Design review of the part built by this model. Coordinates are the model's own, in mm. A direction names the side the tool comes from. Coordinates: 2 decimals unless noted, no trailing zeros. Order: outer loops, then holes, each group sorted by start corner. A loop starts at its lowest first (then second) coordinate and runs counter-clockwise, first axis right, second up. Notation, with made-up numbers: M 55.25,78.5 L 100.25,78.5 A14 ccw 100.25,90.5 Z; hole C 34.5,44.25 d3. An arc over 180 degrees is marked long. Use CSV: the item, a comma, the result in double quotes.
```python
from build123d import *

# Parameters (mm, degrees)
FILLET1_R     = 2.5
CHAMFER1_SIZE = 1


with BuildPart() as part:
    # Sketch1 → Revolve1 (revolve)
    with BuildSketch(Plane.XY, mode=Mode.PRIVATE) as revolve1_sk:
        Polygon((0, 0), (251, 0), (251, 16), (206, 16), (206, 18.5), (170, 18.5), (170, 21), (70, 21), (70, 18.5), (45, 18.5), (45, 16), (0, 16), align=None)
    revolve(revolve1_sk.sketch.rotate(Axis((0, 0, 0), (1, 0, 0)), 90), axis=Axis((0, 0, 0), (1, 0, 0)))

    # Fillet1
    fillet1_edges = [part.edges().sort_by_distance(p)[0] for p in [
        (170, 0, -18.5),
        (70, 0, -18.5),
        (45, 0, -16),
        (206, 0, -16),
    ]]
    fillet(fillet1_edges, radius=FILLET1_R - 0.0001)  # a hair under: the kernel refuses the full size

    # Chamfer1
    chamfer1_edges = [part.edges().sort_by_distance(p)[0] for p in [
        (0, 0, -16),
        (251, 0, -16),
    ]]
    chamfer(chamfer1_edges, length=CHAMFER1_SIZE)


solid = part.part
```
(1) Add section C-C on x = 137.5. State the section outline as (y, z) points.
The answers:
outline,"C 0,0 d42"
(2) Clearance check with flat-ended pins moving along their axes: P1, Ø3, axis at x = 139, y = 9, coming from the +Z side; P2, Ø6, axis at x = 183, y = -12.5, coming from the +Z side; P3, Ø2, axis at x = 112, y = 11, coming from the -Z side. State where each tip first meets the part, or that it passes through.
The answers:
P1,"stops at z = 19.62"
P2,"stops at z = 15.87"
P3,"stops at z = -18.47"
(3) For faces 1 (the face through (189.02, 16.41, 8.54)), 2 (the face through (21.46, 15.62, -3.47)), 3 (the face through (0, 0, 0)), list the 3-axis set-ups (+Z, -Z, +X, -X, +Y, -Y) from which the entire face can be reached by the end or side of a thin tool; tool diameter is ignored.
The answers:
face 1,"+X"
face 2,"-X"
face 3,"+Z, -Z, -X, +Y, -Y"
(4) Wall thickness on probe 1 along Z at (x, y) = (16.5, 0.5); probe 2 along Z at (x, y) = (139, 0.5); probe 3 along Y at (x, z) = (208.5, 14.5): over which ranges is each line inside the solid? List them lowest first.
The answers:
probe 1,"z = -15.99 to 15.99"
probe 2,"z = -20.99 to 20.99"
probe 3,"y = -6.76 to 6.76"
